```python
from build123d import *

# Parameters (mm, degrees)
F0_W      = 120
F0_H      = 75
F1_DEPTH  = 2.5
F2_R      = 7.5
F4_DEPTH  = 2.5
F6_R      = 2.702459
F6_R_2    = 2.81209
F6_R_3    = 2.881868
F6_R_4    = 2.925727
F7_DEPTH  = 2
F5_R      = 1.75775
F5_R_2    = 1.75
F8_DEPTH  = 25
F9_W      = 20
F9_H      = 7
F10_DEPTH = 25


with BuildPart() as f1:
    # F0 (on Top) → F1 (new body)
    with BuildSketch(Plane.XY):
        with Locations((0.016714, -0.087802)):
            Rectangle(F0_W, F0_H)
        Polygon((54.356078, -27.587802), (50.016714, -27.587802), (50.016714, -31.433773), (-49.983286, -31.433773), (-49.983286, -27.587802), (-54.489789, -27.587802), (-54.489789, 27.412198), (-49.983286, 27.412198), (-49.983286, 32.136187), (50.016714, 32.136187), (50.016714, 27.412198), (54.356078, 27.412198), align=None, mode=Mode.SUBTRACT)
    extrude(amount=F1_DEPTH)

    # F2
    f2_edges = [f1.edges().sort_by_distance(p)[0] for p in [
        (-59.983286, 37.412198, 1.25),
        (-59.983286, -37.587802, 1.25),
        (60.016714, -37.587802, 1.25),
        (60.016714, 37.412198, 1.25),
    ]]
    fillet(f2_edges, radius=F2_R)

    # F3 (on Top) → F4 (join)
    with BuildSketch(Plane.XY):
        Polygon((50.016714, -31.433773), (50.016714, -27.587802), (54.356078, -27.587802), (54.356078, 27.412198), (50.016714, 27.412198), (50.016714, 32.136187), (-49.983286, 32.136187), (-49.983286, 27.412198), (-54.489789, 27.412198), (-54.489789, -27.587802), (-49.983286, -27.587802), (-49.983286, -31.433773), align=None)
    extrude(amount=F4_DEPTH)

    # F6 (on face) → F7 (cut)
    with BuildSketch(Plane.XY):
        with Locations((54.343142, -31.448055)):
            Circle(F6_R)
        with Locations((-54.500151, -31.445347)):
            Circle(F6_R_2)
        with Locations((-54.540183, 32.076258)):
            Circle(F6_R_3)
        with Locations((54.324467, 32.097194)):
            Circle(F6_R_4)
    extrude(amount=F7_DEPTH, mode=Mode.SUBTRACT)

    # F5 (on Top) → F8 (cut)
    with BuildSketch(Plane.XY):
        with Locations((-54.489789, 32.136187)):
            Circle(F5_R)
        with Locations((54.356078, 32.136187)):
            Circle(F5_R_2)
        with Locations((54.356078, -31.433773)):
            Circle(F5_R_2)
        with Locations((-54.489789, -31.433773)):
            Circle(F5_R_2)
    extrude(amount=F8_DEPTH, mode=Mode.SUBTRACT)

    # F9 (on face) → F10 (cut)
    with BuildSketch(Plane.XY):
        with Locations((0.016714, 23.912198)):
            Rectangle(F9_W, F9_H)
    extrude(amount=F10_DEPTH, mode=Mode.SUBTRACT)


solid = f1.part
```
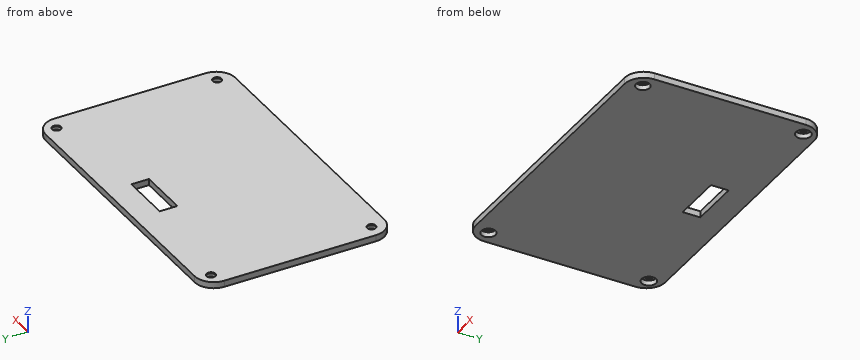
Part model, mm, in its own coordinate system. Give positions to 0.01 mm unless a question says otherwise; leave off trailing zeros. Order: outer loops, then holes, each group sorted by start corner. A loop starts at its lowest first (then second) coordinate and runs counter-clockwise, first axis right, second up. Notation, with made-up numbers: (46.5, 14.25) - (58.5, 14.25) arc R14 cw to (58.5, 18.25) - close; hole circle Ø11 at (64, 31.5). An arc over 180 degrees is marked (long way). Use one line per item in the form item = value.
Item 1: Slice it at A-A on z = 1.5. Give the cut face in (x, y).
Solution:
outline = (-59.98, -30.09) arc R7.5 ccw to (-52.48, -37.59) - (52.52, -37.59) arc R7.5 ccw to (60.02, -30.09) - (60.02, 29.91) arc R7.5 ccw to (52.52, 37.41) - (-52.48, 37.41) arc R7.5 ccw to (-59.98, 29.91) - close; hole circle Ø5.76 at (-54.54, 32.08); hole circle Ø5.62 at (-54.5, -31.45); hole (-9.98, 20.41) - (10.02, 20.41) - (10.02, 27.41) - (-9.98, 27.41) - close; hole circle Ø5.85 at (54.32, 32.1); hole circle Ø5.4 at (54.34, -31.45)
Item 2: Probe probe 1 along Y at (x, z) = (-54.5, 1.2); probe 2 along Y at (x, z) = (-8, 2.45); probe 3 along Y at (x, z) = (-52, 1.1). List the from-to ranges inside material, lowest first. Write a range as from..to.
Solution:
probe_1 = -37.31..-34.26, -28.63..29.19, 34.96..37.14
probe_2 = -37.59..20.41, 27.41..37.41
probe_3 = -37.59..-32.73, -30.16..30.72, 33.44..37.41
Item 3: Pin check, flat tips, straight feed: pin 1 Ø2 at (x, y) = (-54.49, -31.43) entering from +Z; pin 2 Ø3 at (x, y) = (-54, -31) entering from -Z. Stop position of each tip, or through.
Solution:
pin_1 = through
pin_2 = 2
